Check sheet for the modelled part. Datum: model origin and axes. Units: mm. A direction names the side the tool comes from. Round coordinates to 2 decimals unless told otherwise and drop trailing zeros. Order: outer loops, then holes, each group sorted by start corner. A loop starts at its lowest first (then second) coordinate and runs counter-clockwise, first axis right, second up. Notation, with made-up numbers: (86, 47) -> (93, 47) arc R23 ccw to (93, 69) -> close; hole circle Ø8 at (48.5, 49.25). An arc over 180 degrees is marked (long way). Answer in a Markdown table with one row per item.
from build123d import *

# Parameters (mm, degrees)
SKETCH1_R           = 12.5
SKETCH1_R_2         = 2.37125
SKETCH1_R_3         = 1.2
BOSS_EXTRUDE1_DEPTH = 2.715
SKETCH2_R           = 2.15
SKETCH2_R_2         = 3.175
CUT_EXTRUDE1_DEPTH  = 1
CHAMFER1_SIZE       = 0.9
SKETCH3_R           = 3.175
SKETCH3_R_2         = 2.37125
BOSS_EXTRUDE2_DEPTH = 13.81
CUT_EXTRUDE2_START  = -13.81
SKETCH4_R           = 2.67125
SKETCH4_R_2         = 2.37125
CUT_EXTRUDE2_DEPTH  = 13.81
CHAMFER2_SIZE       = 1.482560969
CHAMFER2_SIZE_2     = 1


with BuildPart() as part:
    # Sketch1 → Boss-Extrude1 (new body)
    with BuildSketch(Plane(origin=(0, 0, 0), x_dir=(1, 0, 0), z_dir=(0, 1, 0))):
        with Locations(Location((0, 0, 0), (0, 0, 270))):
            Circle(SKETCH1_R)
        with Locations(Location((0, 0, 0), (0, 0, 270))):
            Circle(SKETCH1_R_2, mode=Mode.SUBTRACT)
        with Locations(Location((0, -6, 0), (0, 0, 270))):
            Circle(SKETCH1_R_3, mode=Mode.SUBTRACT)
        with Locations(Location((-6, 0, 0), (0, 0, 270))):
            Circle(SKETCH1_R_3, mode=Mode.SUBTRACT)
        with Locations(Location((0, 6, 0), (0, 0, 270))):
            Circle(SKETCH1_R_3, mode=Mode.SUBTRACT)
        with Locations(Location((6, 0, 0), (0, 0, 270))):
            Circle(SKETCH1_R_3, mode=Mode.SUBTRACT)
    extrude(amount=BOSS_EXTRUDE1_DEPTH)

    # Sketch2 → Cut-Extrude1 (cut)
    with BuildSketch(Plane(origin=(0, 2.715, 0), x_dir=(1, 0, 0), z_dir=(0, 1, 0))):
        with Locations(Location((0, 6, 0), (0, 0, 270))):
            Circle(SKETCH2_R)
        with Locations(Location((-6, 0, 0), (0, 0, 270))):
            Circle(SKETCH2_R)
        with Locations(Location((6, 0, 0), (0, 0, 270))):
            Circle(SKETCH2_R)
        with Locations(Location((0, -6, 0), (0, 0, 270))):
            Circle(SKETCH2_R)
        with Locations(Location((0, 0, 0), (0, 0, 270))):
            Circle(SKETCH2_R_2)
    extrude(amount=-CUT_EXTRUDE1_DEPTH, mode=Mode.SUBTRACT)

    # Chamfer1
    # the kernel refuses this chamfer: 0.9 mm, written as the material it takes off along each edge
    with BuildSketch(Plane(origin=(0, 1.715, 6), x_dir=(0, 0, 1), z_dir=(1, 0, 0))) as chamfer1_piece_1:
        Polygon((1.2, CHAMFER1_SIZE), (1.2 + CHAMFER1_SIZE, 0), (1.2, 0), align=None)
    revolve(axis=Axis((0, 1.715, 6), (0, -1, 0)), mode=Mode.SUBTRACT)
    with BuildSketch(Plane(origin=(6, 1.715, 0), x_dir=(0, 0, 1), z_dir=(1, 0, 0))) as chamfer1_piece_2:
        Polygon((1.2, CHAMFER1_SIZE), (1.2 + CHAMFER1_SIZE, 0), (1.2, 0), align=None)
    revolve(axis=Axis((6, 1.715, 0), (0, -1, 0)), mode=Mode.SUBTRACT)
    with BuildSketch(Plane(origin=(0, 1.715, 0), x_dir=(0, 0, 1), z_dir=(1, 0, 0))) as chamfer1_piece_3_section:
        Polygon((2.37125, CHAMFER1_SIZE), (2.37125 + CHAMFER1_SIZE, 0), (2.37125, 0), align=None)
    chamfer1_piece_3 = revolve(axis=Axis((0, 1.715, 0), (0, -1, 0)), mode=Mode.PRIVATE)
    chamfer1_piece_3 = chamfer1_piece_3 & Plane(origin=(0, 1.217857085, 0), x_dir=(0, 0, 1), z_dir=(0, 1, 0)) * Cylinder(3.175, 14, mode=Mode.PRIVATE)
    add(chamfer1_piece_3, mode=Mode.SUBTRACT)
    with BuildSketch(Plane(origin=(-6, 1.715, 0), x_dir=(0, 0, 1), z_dir=(1, 0, 0))) as chamfer1_piece_4:
        Polygon((1.2, CHAMFER1_SIZE), (1.2 + CHAMFER1_SIZE, 0), (1.2, 0), align=None)
    revolve(axis=Axis((-6, 1.715, 0), (0, -1, 0)), mode=Mode.SUBTRACT)
    with BuildSketch(Plane(origin=(0, 1.715, -6), x_dir=(0, 0, 1), z_dir=(1, 0, 0))) as chamfer1_piece_5:
        Polygon((1.2, CHAMFER1_SIZE), (1.2 + CHAMFER1_SIZE, 0), (1.2, 0), align=None)
    revolve(axis=Axis((0, 1.715, -6), (0, -1, 0)), mode=Mode.SUBTRACT)

    # Sketch3 → Boss-Extrude2 (add)
    with BuildSketch(Plane.XZ):
        with Locations(Location((0, 0, 0), (0, 0, 270))):
            Circle(SKETCH3_R)
        with Locations(Location((0, 0, 0), (0, 0, 270))):
            Circle(SKETCH3_R_2, mode=Mode.SUBTRACT)
    extrude(amount=-BOSS_EXTRUDE2_DEPTH)

    # Sketch4 → Cut-Extrude2 (cut)
    with BuildSketch(Plane(origin=(0, 13.81, 0), x_dir=(1, 0, 0), z_dir=(0, 1, 0)).offset(CUT_EXTRUDE2_START)):
        with Locations(Location((0, 0, 0), (0, 0, 270))):
            Circle(SKETCH4_R)
        Circle(SKETCH4_R_2, mode=Mode.SUBTRACT)
    extrude(amount=CUT_EXTRUDE2_DEPTH, mode=Mode.SUBTRACT)

    # Chamfer2
    # the kernel refuses this chamfer: 1.482560969, 1 mm, written as the material it takes off along each edge
    with BuildSketch(Plane(origin=(0, 13.81, 0), x_dir=(0, 0, -1), z_dir=(-1, 0, 0))) as chamfer2_piece_1:
        Polygon((3.175, CHAMFER2_SIZE), (3.175 - CHAMFER2_SIZE_2, 0), (3.175, 0), align=None)
    revolve(axis=Axis((0, 13.81, 0), (0, -1, 0)), mode=Mode.SUBTRACT)


solid = part.part
Item 1: Cross-section at A-A (z = 0). State how many separate pieces and enclosed holes the cut face has, and give its area (3 significant figures).
Result sheet:
| item | result |
|---|---|
| separate pieces | 4 |
| enclosed holes | 0 |
| area | 45.0 mm^2 |
Item 2: Mould release check, pull along Z, two halves, no side actions. Record for faces 3 (the cylindrical face through (7.19, 0.4, -0.16)), 4 (the flat face through (3, 0, 0)), 5 (the cylindrical face through (0.09, 2.22, 3.85)), 6 (the cylindrical face through (3.755, 1.338, 11.923)): pulls with the +Z half, pulls with the -Z half, needs draft (parallel to the pull), parting line crosses it, or undercut.
Result sheet:
| item | result |
|---|---|
| face 3 | undercut |
| face 4 | needs draft |
| face 5 | undercut |
| face 6 | parting line crosses it |
Item 3: Depth check by flat-ended pin: P1, Ø3.5, axis at x = -0.5, z = -5.5, coming from the +Y side (3 decimals); P2, Ø3, axis at x = 0, z = -6, coming from the +Y side (3 decimals); P3, Ø4, axis at x = 8, z = -7, coming from the -Y side; P4, Ø1.5, axis at y = 4.5, z = 1, coming from the +X side. Enter the tip coordinate at first touch or a pass-through.
Result sheet:
| item | result |
|---|---|
| P1 | stops at y = 2.715 |
| P2 | stops at y = 1.115 |
| P3 | stops at y = 0 |
| P4 | stops at x = 3.17 |
Item 4: Scan lines: line 1 (X direction, y = 0.3, z = 0); line 2 (X direction, y = 2, z = 0); line 3 (X direction, y = 3.75, z = 0) (3 decimals). Record each from-to range of solid material in increasing order. Write a range as [from, to].
Result sheet:
| item | result |
|---|---|
| line 1 | x = [-12.5, -7.2], [-4.8, -2.67], [2.67, 4.8], [7.2, 12.5] |
| line 2 | x = [-12.5, -8.15], [-3.85, -2.67], [2.67, 3.85], [8.15, 12.5] |
| line 3 | x = [-3.175, -2.671], [2.671, 3.175] |
Item 5: Set-up check for faces 1 (the cylindrical face through (2.65, 6.45, -0.35)), 2 (the cylindrical face through (-1.93, 7.45, 2.52)): record each of +Z, -Z, +X, -X, +Y, -Y from which the full face is reachable in a straight line by a thin tool's end or side.
Result sheet:
| item | result |
|---|---|
| face 1 | +Y, -Y |
| face 2 | +Y |
Item 6: Cross-section at D-D (z = 6). Record the boundary of the cut face in (x, y) (3 decimals), and give its area (3 significant figures).
Result sheet:
| item | result |
|---|---|
| outline | (-10.966, 0) -> (-1.2, 0) -> (-1.2, 0.815) -> (-2.1, 1.715) -> (-2.15, 1.715) -> (-2.15, 2.715) -> (-10.966, 2.715) -> close; (1.2, 0) -> (10.966, 0) -> (10.966, 2.715) -> (2.15, 2.715) -> (2.15, 1.715) -> (2.1, 1.715) -> (1.2, 0.815) -> close |
| area | 50.3 mm^2 |
